Read the model definition and answer for the solid it produces. Units are mm, in the model's axes. Face numbers are marked on the shaded views. A direction names the side the tool comes from. Coordinates: 2 decimals unless noted, no trailing zeros. Write each loop counter-clockwise with the first axis right and the second up, starting at its lowest first coordinate (ties: lowest second). Pieces come first, ordered by that corner, then holes.
1) The part is cut by section D-D (y = -4). Determine the outline of the cut face in (x, z), then the cut area to 3 significant figures.
2) Determine the mould class of the marked faces 1, 2 and 3 for opening direction Z: +Z half, -Z half, draft (parallel to the pull), parting line (faces both ways), or undercut.
3) The part is cut by section C-C (z = 0). Determine the outline of the cut face in (x, y), then the cut area to 3 significant figures.
4) The part is cut by section A-A (y = 7.25). Determine the outline of the cut face in (x, z).
5) Find the intervals of material crossed by line 1 (X direction, y = 13.25, z = -29); line 2 (Z direction, x = -6, y = -8); line 3 (Z direction, x = -9, y = 7), in increasing order.
6) Each of these flat-tipped pins is pushed along its axis until it touches: pin 1 Ø5 at (x, z) = (0, 1) entering from -Y; pin 2 Ø2 at (x, z) = (4.5, -28) entering from -Y; pin 3 Ø3 at (x, y) = (2.5, 7) entering from +Z. Where does it stop, or does it pass through?
7) Which of the six approach directions +Z, -Z, +X, -X, +Y, -Y give full straight-line access (tool end or side, diameter ignored) to the marked faces 4, 5 and 6?
8) The part is cut by section B-B (x = 0). Determine the outline of the cut face in (y, z), then the cut area to 3 significant figures.
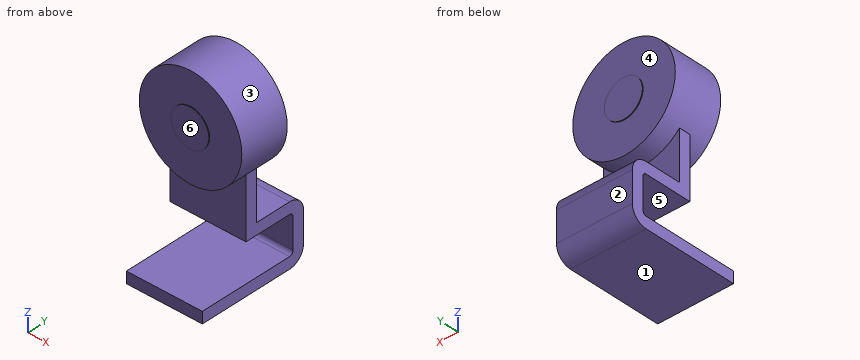
from build123d import *

# Parameters (mm, degrees)
F0_R     = 13.5
F0_R_2   = 5
F1_DEPTH = 6.5
F2_DEPTH = 6.7
F3_R     = 5
F4_DEPTH = 1.5
F6_DEPTH = 10


with BuildPart() as f1:
    # F0 (on Front) → F1 (new body, symmetric)
    with BuildSketch(Plane.XZ):
        Circle(F0_R)
        Circle(F0_R_2, mode=Mode.SUBTRACT)
    extrude(amount=F1_DEPTH, both=True)

    # F0 (on Front) → F2 (join, symmetric)
    with BuildSketch(Plane.XZ):
        Circle(F0_R_2)
    extrude(amount=F2_DEPTH, both=True)

    # F3 (on Front) → F4 (join, symmetric)
    with BuildSketch(Plane.XZ):
        with BuildLine():
            Line((10, -25), (10, 0))
            ThreePointArc((10, 0), (0, 10), (-10, 0))
            Line((-10, 0), (-10, -25))
            Line((-10, -25), (10, -25))
        make_face()
        Circle(F3_R, mode=Mode.SUBTRACT)
    extrude(amount=F4_DEPTH, both=True)

    # F5 (on Right) → F6 (join, symmetric)
    with BuildSketch(Plane.YZ):
        with BuildLine():
            Line((0, -22), (0, -25))
            Line((0, -25), (1.5, -25))
            Line((1.5, -25), (11, -25))
            ThreePointArc((11, -25), (11.7071067812, -25.2928932188), (12, -26))
            Line((12, -26), (12, -34))
            ThreePointArc((12, -34), (11.7071067812, -34.7071067812), (11, -35))
            Line((11, -35), (-14, -35))
            Line((-14, -35), (-14, -38))
            Line((-14, -38), (11, -38))
            ThreePointArc((11, -38), (13.8284271247, -36.8284271247), (15, -34))
            Line((15, -34), (15, -26))
            ThreePointArc((15, -26), (13.8284271247, -23.1715728753), (11, -22))
            Line((11, -22), (0, -22))
        make_face()
    extrude(amount=F6_DEPTH, both=True)


solid = f1.part
Reported:
1. outline: circle Ø27 at (0, 0); (-10, -38) - (10, -38) - (10, -35) - (-10, -35) - close
1. area: 633 mm2
2. face 1: -Z half
2. face 2: draft
2. face 3: undercut
3. outline: (-13.5, -6.5) - (-5, -6.5) - (-5, -6.7) - (5, -6.7) - (5, -6.5) - (13.5, -6.5) - (13.5, 6.5) - (5, 6.5) - (5, 6.7) - (-5, 6.7) - (-5, 6.5) - (-13.5, 6.5) - close
3. area: 355 mm2
4. outline: (-10, -38) - (10, -38) - (10, -35) - (-10, -35) - close; (-10, -25) - (10, -25) - (10, -22) - (-10, -22) - close
5. line 1: x = -10 to 10
5. line 2: z = -38 to -35
5. line 3: z = -38 to -35, -25 to -22
6. pin 1: stops at y = -6.7
6. pin 2: stops at y = 12
6. pin 3: stops at z = 13.46
7. face 4: +Y
7. face 5: +X, -X, -Y
7. face 6: +Z, +X, -X, -Y
8. outline: (-14, -38) - (11, -38) arc R4 ccw to (15, -34) - (15, -26) arc R4 ccw to (11, -22) - (1.5, -22) - (1.5, -13.5) - (6.5, -13.5) - (6.5, -5) - (6.7, -5) - (6.7, 5) - (6.5, 5) - (6.5, 13.5) - (-6.5, 13.5) - (-6.5, 5) - (-6.7, 5) - (-6.7, -5) - (-6.5, -5) - (-6.5, -13.5) - (-1.5, -13.5) - (-1.5, -25) - (11, -25) arc R1 cw to (12, -26) - (12, -34) arc R1 cw to (11, -35) - (-14, -35) - close
8. area: 541 mm2
